Design review of the part built by this model. Coordinates are the model's own, in mm. A direction names the side the tool comes from. Round coordinates to 2 decimals unless told otherwise and drop trailing zeros. Order: outer loops, then holes, each group sorted by start corner. A loop starts at its lowest first (then second) coordinate and runs counter-clockwise, first axis right, second up. Notation, with made-up numbers: (85, -3) - (123, -3) arc R23 ccw to (123, 24) - close; hole circle Ø7 at (5, 30.25). An arc over 180 degrees is marked (long way). Use CSV: the item, a comma, the result in double quotes.
from build123d import *

# Parameters (mm, degrees)
SKETCH_1_W          = 24.3
SKETCH_1_H          = 3
EXTRUDE_1_DEPTH     = 5
EXTRUDE_1_2_DEPTH   = 5
SKETCH_2_W          = 24.3
SKETCH_2_H          = 18
EXTRUDE_2_DEPTH     = 3
EXTRUDE_3_DEPTH     = 2
EXTRUDE_5_DEPTH     = 6
SKETCH_7_W          = 2
SKETCH_7_H          = 8
EXTRUDE_6_DEPTH     = 26.3
SKETCH_8_R          = 2.5
CUT_EXTRUDE_2_DEPTH = 2


with BuildPart() as part:
    # Sketch 1 → Extrude 1 (new body)
    with BuildSketch(Plane.XY):
        with Locations((0, 7.5)):
            Rectangle(SKETCH_1_W, SKETCH_1_H)
    extrude(amount=EXTRUDE_1_DEPTH)



with BuildPart() as body_2:
    # Sketch 1 → Extrude 1 2 (new body)
    with BuildSketch(Plane.XY):
        with Locations((0, -7.5)):
            Rectangle(SKETCH_1_W, SKETCH_1_H)
    extrude(amount=EXTRUDE_1_2_DEPTH)


with BuildPart() as body_3:
    # Sketch 2 → Extrude 2 (new body)
    with BuildSketch(Plane(origin=(0, 0, 0), x_dir=(-1, 0, 0), z_dir=(0, 0, -1))):
        Rectangle(SKETCH_2_W, SKETCH_2_H)
    extrude(amount=EXTRUDE_2_DEPTH)


with BuildPart() as part_1:
    add(part.part)

    add(body_2.part)  # Extrude 3 merges body 2

    add(body_3.part)  # Extrude 3 merges body 3
    # Sketch 3 → Extrude 3 (add)
    with BuildSketch(Plane(origin=(12.15, 0, 0), x_dir=(0, 0, -1), z_dir=(1, 0, 0))):
        Polygon((-5, 6), (-5, 9), (3, 9), (3, -9), (-5, -9), (-5, -6), (-2, -6), (0, -4), (0, 4), (-2, 6), align=None)
    extrude(amount=EXTRUDE_3_DEPTH)

    # Sketch 6 → Extrude 5 (add)
    with BuildSketch(Plane(origin=(14.15, 0, 0), x_dir=(0, 0, -1), z_dir=(1, 0, 0))):
        with BuildLine():
            Line((7.6583166, 1.870824966), (3, 6))
            Line((3, 6), (3, 0))
            Line((3, 0), (3.5, 0))
            ThreePointArc((3.5, 0), (4.974278668, 2.279889416), (7.6583166, 1.870824966))
        make_face()
        with BuildLine():
            ThreePointArc((8.5, 0), (8.279889416, 1.025721332), (7.6583166, 1.870824966))
            ThreePointArc((7.6583166, 1.870824966), (4.974278668, 2.279889416), (3.5, 0))
            Line((3.5, 0), (4.5, 0))
            ThreePointArc((4.5, 0), (6, 1.5), (7.5, 0))
            Line((7.5, 0), (8.5, 0))
        make_face()
        with BuildLine():
            ThreePointArc((7.6583166, -1.870824966), (8.279889416, -1.025721332), (8.5, 0))
            Line((8.5, 0), (7.5, 0))
            ThreePointArc((7.5, 0), (6, -1.5), (4.5, 0))
            Line((4.5, 0), (3.5, 0))
            ThreePointArc((3.5, 0), (4.974278668, -2.279889416), (7.6583166, -1.870824966))
        make_face()
        with BuildLine():
            Line((3.5, 0), (3, 0))
            Line((3, 0), (3, -6))
            Line((3, -6), (7.6583166, -1.870824966))
            ThreePointArc((7.6583166, -1.870824966), (4.974278668, -2.279889416), (3.5, 0))
        make_face()
    extrude(amount=-EXTRUDE_5_DEPTH)

    # Sketch 7 → Extrude 6 (add)
    with BuildSketch(Plane(origin=(14.15, 0, 0), x_dir=(0, 0, -1), z_dir=(1, 0, 0))):
        with Locations((-4, 13)):
            Rectangle(SKETCH_7_W, SKETCH_7_H)
        with Locations((-4, -13)):
            Rectangle(SKETCH_7_W, SKETCH_7_H)
    extrude(amount=-EXTRUDE_6_DEPTH)

    # Sketch 8 → Cut-Extrude 2 (cut)
    with BuildSketch(Plane(origin=(0, 0, 3), x_dir=(-1, 0, 0), z_dir=(0, 0, -1))):
        with Locations((5.85, -13)):
            Circle(SKETCH_8_R)
        with Locations((-9.15, -13)):
            Circle(SKETCH_8_R)
        with Locations((-9.15, 13)):
            Circle(SKETCH_8_R)
        with Locations((5.85, 13)):
            Circle(SKETCH_8_R)
    extrude(amount=-CUT_EXTRUDE_2_DEPTH, mode=Mode.SUBTRACT)


solid = part_1.part
1) For faces 1 (the face through (8.15, 0, -4)), 2 (the face through (13, -5, 1)), 3 (the face through (9.69, 10.56, 3.99)), 4 (the face through (1, -17, 4)), 5 (the face through (12.15, 5.2, 0.8)), list the 3-axis set-ups (+Z, -Z, +X, -X, +Y, -Y) from which the entire face can be reached by the end or side of a thin tool; tool diameter is ignored.
Data:
face 1,"-Z, -X, +Y, -Y"
face 2,"+Z, +X, -X"
face 3,"+Z, -Z"
face 4,"+Z, -Z, +X, -X, -Y"
face 5,"+Z, -X"
2) We need section D-D (x = 4). Give the boundary of the cut face in (y, z), then the cut area to 3 significant figures.
Data:
outline,"(-17, 3) - (-9, 3) - (-9, -3) - (9, -3) - (9, 3) - (17, 3) - (17, 5) - (6, 5) - (6, 0) - (-6, 0) - (-6, 5) - (-17, 5) - close"
area,"116 mm2"
3) Insertion check: pin 1 Ø6 at (x, z) = (0.5, -1) entering from -Y; pin 2 Ø14.5 at (x, y) = (3.5, -2) entering from -Z; pin 3 Ø6 at (x, y) = (9.15, 13) entering from -Z; pin 4 Ø0.6 at (y, z) = (5.5, 1) entering from -X. Each pin has a flat end and moves straight along its axis. Give the tip position at first contact, or say it passes through.
Data:
pin 1,"stops at y = -9"
pin 2,"stops at z = -8.5"
pin 3,"stops at z = 3"
pin 4,"stops at x = 12.15"
4) We need section A-A (x = 9.15). Give the boundary of the cut face in (y, z), then the cut area to 3 significant figures.
Data:
outline,"(-17, 3) - (-15.5, 3) - (-15.5, 5) - (-17, 5) - close; (-10.5, 3) - (-9, 3) - (-9, -3) - (-6, -3) - (-1.87, -7.66) arc R2.5 ccw to (1.87, -7.66) - (6, -3) - (9, -3) - (9, 3) - (10.5, 3) - (10.5, 5) - (6, 5) - (6, 0) - (-6, 0) - (-6, 5) - (-10.5, 5) - close; (15.5, 3) - (17, 3) - (17, 5) - (15.5, 5) - close; hole circle Ø3 at (0, -6)"
area,"128 mm2"
5) To check wall thickness, follow L1, parallel to Y at x = 9.15, z = 3.8; L2, parallel to Z at x = 9.25, y = 0; L3, parallel to Y at x = 11, z = 4. State the ranges of each line that lie inside material, in increasing order. Write a range as from..to.
Data:
L1,"y = -17..-15.5, -10.5..-6, 6..10.5, 15.5..17"
L2,"z = -8.5..-7.5, -4.5..0"
L3,"y = -17..-14.68, -11.32..-6, 6..11.32, 14.68..17"
6) We need section B-B (y = 11.5). Give the boundary of the cut face in (x, z), then the cut area to 3 significant figures.
Data:
outline,"(-12.15, 3) - (-7.85, 3) - (-7.85, 5) - (-12.15, 5) - close; (-3.85, 3) - (7.15, 3) - (7.15, 5) - (-3.85, 5) - close; (11.15, 3) - (14.15, 3) - (14.15, 5) - (11.15, 5) - close"
area,"36.6 mm2"
7) The part is to be moulded in two halves that separate along Y. For faces 6 (the face through (11.2, 0.9, -4.8)), 7 (the face through (1, 9, 0)), 8 (the face through (1, -9, 0)), 9 (the face through (1, -6, 3)), say which applies: +Y half, -Y half, draft (parallel to the pull), parting line (faces both ways), or undercut.
Data:
face 6,"undercut"
face 7,"+Y half"
face 8,"-Y half"
face 9,"undercut"
8) We need section C-C (z = -6.5). Give the boundary of the cut face in (x, y).
Data:
outline,"(8.15, -2.9) - (14.15, -2.9) - (14.15, -1.41) - (8.15, -1.41) - close; (8.15, 1.41) - (14.15, 1.41) - (14.15, 2.9) - (8.15, 2.9) - close"
